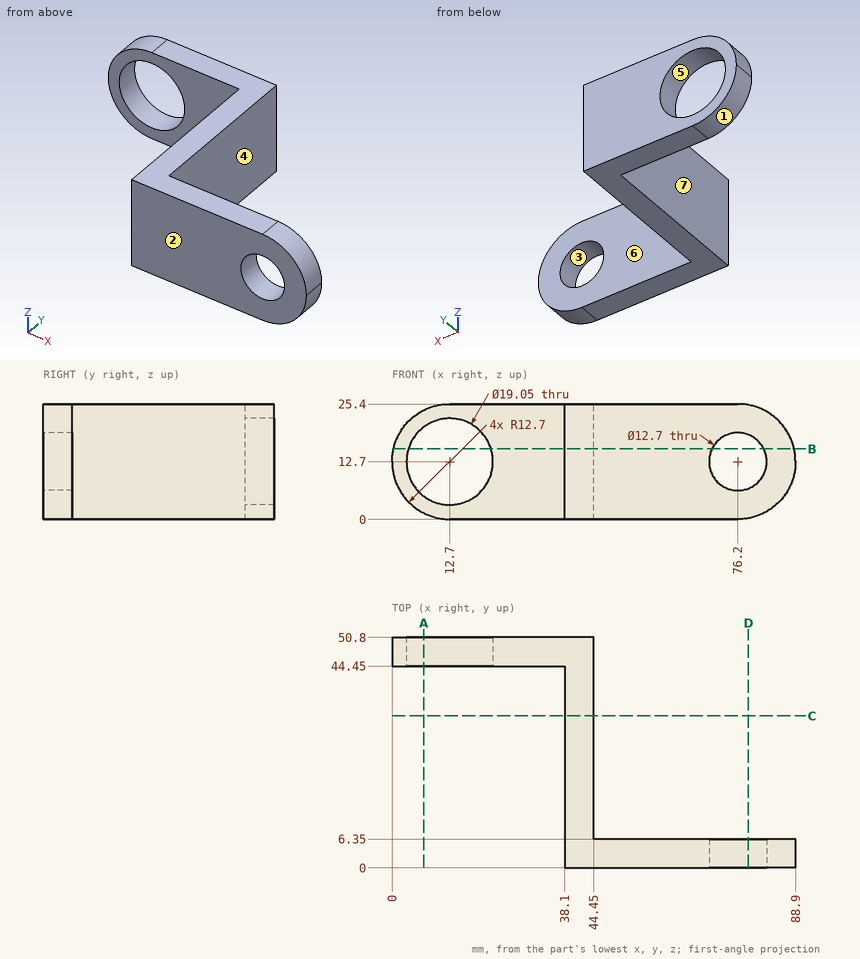
Verification items for this drawing (mm, ordinates from the low corner). A direction names the side the tool comes from. Give positions to 0.01 mm unless a question says otherwise; leave off trailing zeros. Write each loop counter-clockwise with the first axis right and the second up, starting at its lowest first coordinate (ties: lowest second). Pieces come first, ordered by that corner, then holes.
1) Release check for a two-part mould opening along X. For the marked faces 1, 2, 3 and 4 record: pulls with the +X half, pulls with the -X half, needs draft (parallel to the pull), parting line crosses it, or undercut.
2) Section check D-D, the plane x = 78.5. Record the boundary of the cut face in (y, z).
3) Section check A-A, the plane x = 7. Record the boundary of the cut face in (y, z), and give its area (3 significant figures).
4) Material ranges on L1, parallel to Z at x = 76, y = 4; L2, parallel to Z at x = 12.7, y = 48.75 (3 decimals); L3, parallel to Y at x = 23, z = 8, recorded low to high.
5) Gauge pin test, flat ends, axial feed: pin 1 (3 mm diameter, centred on y = 42.5, z = 12.5, fed in from +X); pin 2 (2 mm diameter, centred on y = 12.5, z = 14, fed in from -X); pin 3 (2 mm diameter, centred on x = 46.5, z = 16, fed in from +Y). Record the tip position at first contact, or that the pin passes through.
6) Access from +Z, -Z, +X, -X, +Y, -Y to the whole of each face (thin tool, end or side, straight path). Record for the marked faces 5, 6 and 7.
7) Section check C-C, the plane y = 33.5. Record the boundary of the cut face in (x, z), and give its area (3 significant figures).
8) Section check B-B, the plane z = 15.5. Record the boundary of the cut face in (x, y), and give its area (3 significant figures).
Computed:
1. face 1: pulls with the -X half
1. face 2: needs draft
1. face 3: undercut
1. face 4: pulls with the +X half
2. outline: (0, 0.21) - (6.35, 0.21) - (6.35, 6.78) - (0, 6.78) - close; (0, 18.62) - (6.35, 18.62) - (6.35, 25.19) - (0, 25.19) - close
3. outline: (44.45, 1.35) - (50.8, 1.35) - (50.8, 5.07) - (44.45, 5.07) - close; (44.45, 20.33) - (50.8, 20.33) - (50.8, 24.05) - (44.45, 24.05) - close
3. area: 47.2 mm2
4. L1: z = 0 to 6.35, 19.05 to 25.4
4. L2: z = 0 to 3.175, 22.225 to 25.4
4. L3: y = 44.45 to 50.8
5. pin 1: stops at x = 44.45
5. pin 2: stops at x = 38.1
5. pin 3: stops at y = 6.35
6. face 5: +Y, -Y
6. face 6: +Z, -Z, +X, +Y
6. face 7: +Z, -Z, -X, -Y
7. outline: (38.1, 0) - (44.45, 0) - (44.45, 25.4) - (38.1, 25.4) - close
7. area: 161 mm2
8. outline: (0.31, 44.45) - (3.6, 44.45) - (3.6, 50.8) - (0.31, 50.8) - close; (21.8, 44.45) - (38.1, 44.45) - (38.1, 0) - (70.5, 0) - (70.5, 6.35) - (44.45, 6.35) - (44.45, 50.8) - (21.8, 50.8) - close; (81.9, 0) - (88.59, 0) - (88.59, 6.35) - (81.9, 6.35) - close
8. area: 655 mm2
